```python
from build123d import *

# Parameters (mm, degrees)
SKETCH1_W           = 20
SKETCH1_H           = 50
BOSS_EXTRUDE1_DEPTH = 3
SKETCH2_R           = 5.1
SKETCH2_R_2         = 1.75
SKETCH2_R_3         = 2
CUT_EXTRUDE1_DEPTH  = 28.092434368
FILLET1_R           = 5


with BuildPart() as part:
    # Sketch1 → Boss-Extrude1 (new body)
    with BuildSketch(Plane(origin=(0, 0, 0), x_dir=(1, 0, 0), z_dir=(0, 1, 0))):
        Rectangle(SKETCH1_W, SKETCH1_H)
    extrude(amount=BOSS_EXTRUDE1_DEPTH)

    # Sketch2 → Cut-Extrude1 (cut, through all)
    with BuildSketch(Plane(origin=(0, 3, 0), x_dir=(1, 0, 0), z_dir=(0, 1, 0))):
        with Locations(Location((0, 10, 0), (0, 0, 270))):
            Circle(SKETCH2_R)
        with Locations(Location((0, 18, 0), (0, 0, 270))):
            Circle(SKETCH2_R_2)
        with Locations(Location((0, 2, 0), (0, 0, 270))):
            Circle(SKETCH2_R_2)
        with Locations(Location((0, -10, 0), (0, 0, 270))):
            Circle(SKETCH2_R_3)
        with Locations(Location((0, -20, 0), (0, 0, 270))):
            Circle(SKETCH2_R_3)
    extrude(amount=-CUT_EXTRUDE1_DEPTH, mode=Mode.SUBTRACT)

    # Fillet1
    fillet1_edges = [part.edges().sort_by_distance(p)[0] for p in [
        (10, 1.5, 25),
        (-10, 1.5, 25),
        (-10, 1.5, -25),
        (10, 1.5, -25),
    ]]
    fillet(fillet1_edges, radius=FILLET1_R)


solid = part.part
```
Work out the finished part from the listing and answer in its coordinate system (mm). Give positions to 0.01 mm unless a question says otherwise; leave off trailing zeros. Loops run counter-clockwise (first coordinate to the right, second up) from the corner with the lowest first, then second, coordinate; pieces in that order, holes last. Notation, with made-up numbers: M 84,61.25 L 103,61.25 A19 ccw 103,71.25 Z; hole C 84.25,29 d6. An arc over 180 degrees is marked long. One line per item, written item: value. Start each with the question number.
1. Find section A-A (z = -10). Give the vertices of the cut face in (x, y).
2. Find section B-B (x = 0). Give the vertices of the cut face in (y, z).
3. Find the intervals of material crossed by probe 1 along X at (y, z) = (0.65, 10); probe 2 along X at (y, z) = (1.75, -10); probe 3 along Z at (x, y) = (-1, 1), in increasing order.
4. Find section D-D (x = 3.25). Give the vertices of the cut face in (y, z), and give its area (3 significant figures).
5. Find section C-C (y = 2.05). Give the vertices of the cut face in (x, z).
6. Determine the mould class of faces 1 (the face through (8, 2, -24)), 2 (the face through (0.08, 1.52, -19.75)), 3 (the face through (1.532, 1.521, -5.136)), 4 (the face through (-10, 1, 0)) for opening direction X: released by +X, released by -X, zero draft, split by the parting line, or undercut.
Reported:
1. outline: M -10,0 L -5.1,0 L -5.1,3 L -10,3 Z; M 5.1,0 L 10,0 L 10,3 L 5.1,3 Z
2. outline: M 0,-25 L 3,-25 L 3,-19.75 L 0,-19.75 Z; M 0,-16.25 L 3,-16.25 L 3,-15.1 L 0,-15.1 Z; M 0,-4.9 L 3,-4.9 L 3,-3.75 L 0,-3.75 Z; M 0,-0.25 L 3,-0.25 L 3,8 L 0,8 Z; M 0,12 L 3,12 L 3,18 L 0,18 Z; M 0,22 L 3,22 L 3,25 L 0,25 Z
3. probe 1: x = -10 to -2, 2 to 10
3. probe 2: x = -10 to -5.1, 5.1 to 10
3. probe 3: z = -25 to -19.44, -16.56 to -15, -5 to -3.44, -0.56 to 8.27, 11.73 to 18.27, 21.73 to 25
4. outline: M 0,-25 L 3,-25 L 3,-13.93 L 0,-13.93 Z; M 0,-6.07 L 3,-6.07 L 3,25 L 0,25 Z
4. area: 126 mm²
5. outline: M -10,-20 A5 ccw -5,-25 L 5,-25 A5 ccw 10,-20 L 10,20 A5 ccw 5,25 L -5,25 A5 ccw -10,20 Z; hole C 0,-10 d10.2; hole C 0,10 d4; hole C 0,20 d4; hole C 0,-18 d3.5; hole C 0,-2 d3.5
6. face 1: released by +X
6. face 2: undercut
6. face 3: undercut
6. face 4: released by -X
